The drawing under review shows one solid part. Ordinate dimensions are in mm from its lowest x, y, z. A direction names the side the tool comes from. Round coordinates to 2 decimals unless told otherwise and drop trailing zeros. Write each loop counter-clockwise with the first axis right and the second up, starting at its lowest first coordinate (ties: lowest second). Pieces come first, ordered by that corner, then holes. Notation, with made-up numbers: (-8.75, 26.25) - (49.25, 26.25) arc R19 cw to (49.25, 54.25) - close; hole circle Ø4 at (43.5, 71). An arc over 180 degrees is marked (long way). Answer in a Markdown table with one row per item. Add a question column.
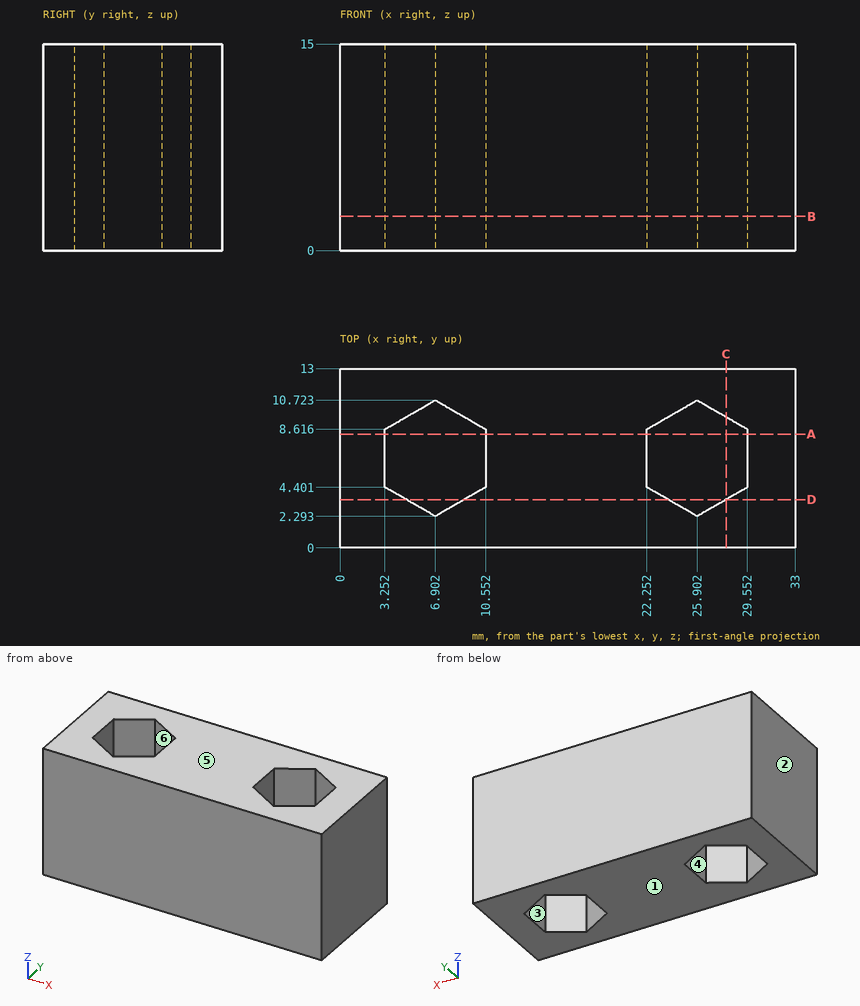
Q1. Add section A-A on y = 8.25. State the section outline as (x, z) points.
Q2. Add section D-D on y = 3.5. State the section outline as (x, z) points.
Q3. To check wall thickness, follow probe 1 along X at (y, z) = (7, 13); probe 2 along X at (y, z) = (9, 4.5) (1 decimal); probe 3 along Y at (x, z) = (5, 12.25) (1 decimal). State the ranges of each line that lie inside material, in increasing order.
Q4. Draft analysis for pull direction X (two halves, no side actions). For the marked faces 1, 2, 3 and 4, state which applies: released by +X, released by -X, zero draft, split by the parting line, or undercut.
Q5. Insertion check: pin 1 Ø1 at (x, z) = (24, 8.5) entering from -Y. The pin has a flat end and moves straight along its axis. Give the tip position at first contact, or say it passes through.
Q6. Add section C-C on x = 28. State the section outline as (y, z) points (1 decimal), then the cut area to 3 significant figures.
Q7. Add section B-B on z = 2.5. State the section outline as (x, y) points (1 decimal), then the cut area to 3 significant figures.
Q8. Tool access review of the marked faces 5 and 6: name each direction out of +Z, -Z, +X, -X, +Y, -Y from which nothing blocks a thin tool from reaching the whole face with its end or side.
Answer sheet:
| question | item | result |
|---|---|---|
| 1 | outline | (0, 0) - (3.25, 0) - (3.25, 15) - (0, 15) - close; (10.55, 0) - (22.25, 0) - (22.25, 15) - (10.55, 15) - close; (29.55, 0) - (33, 0) - (33, 15) - (29.55, 15) - close |
| 2 | outline | (0, 0) - (4.81, 0) - (4.81, 15) - (0, 15) - close; (8.99, 0) - (23.81, 0) - (23.81, 15) - (8.99, 15) - close; (27.99, 0) - (33, 0) - (33, 15) - (27.99, 15) - close |
| 3 | probe 1 | x = 0 to 3.25, 10.55 to 22.25, 29.55 to 33 |
| 3 | probe 2 | x = 0 to 3.9, 9.9 to 22.9, 28.9 to 33 |
| 3 | probe 3 | y = 0 to 3.4, 9.6 to 13 |
| 4 | face 1 | zero draft |
| 4 | face 2 | released by -X |
| 4 | face 3 | undercut |
| 4 | face 4 | undercut |
| 5 | pin 1 | stops at y = 0 |
| 6 | outline | (0, 0) - (3.5, 0) - (3.5, 15) - (0, 15) - close; (9.5, 0) - (13, 0) - (13, 15) - (9.5, 15) - close |
| 6 | area | 105 mm² |
| 7 | outline | (0, 0) - (33, 0) - (33, 13) - (0, 13) - close; hole (3.3, 4.4) - (6.9, 2.3) - (10.6, 4.4) - (10.6, 8.6) - (6.9, 10.7) - (3.3, 8.6) - close; hole (22.3, 4.4) - (25.9, 2.3) - (29.6, 4.4) - (29.6, 8.6) - (25.9, 10.7) - (22.3, 8.6) - close |
| 7 | area | 337 mm² |
| 8 | face 5 | +Z, +X, -X, +Y, -Y |
| 8 | face 6 | +Z, -Z |
